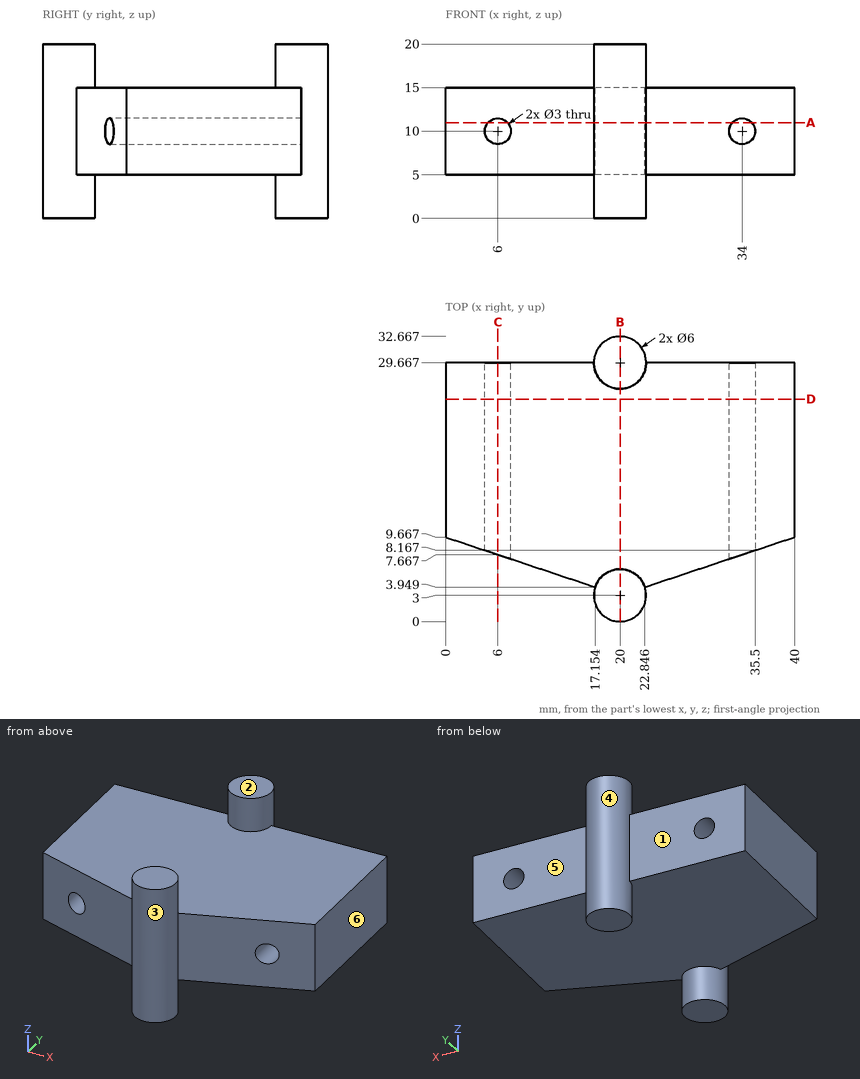
Can you work these out from the drawing? Everything is in mm from the part's minimum corner. A direction names the side the tool comes from. Coordinates: 2 decimals unless noted, no trailing zeros. Loops run counter-clockwise (first coordinate to the right, second up) from the corner with the lowest first, then second, coordinate; pieces in that order, holes last. Notation, with made-up numbers: (-36.75, -8.5) - (10.25, -8.5) arc R16 cw to (10.25, 18.5) - close; hole circle Ø6 at (65.5, 14.5). An arc over 180 degrees is marked (long way). Put each result on its own line as item: value. Start each with the question number.
Item 1: If we mould it in two halves opening along Y, with no side actions, what happens to the marked faces 1, 2 and 3? For each: +Y half, -Y half, draft (parallel to the pull), parting line (faces both ways), or undercut.
Item 2: If I drill on line 1 along X through (y, z) = (21.5, 10); line 2 along Z through (x, y) = (34, 18); line 3 along Z through (x, y) = (4, 9.5), over which ranges is the centre line in solid material (lowest first)?
Item 3: Suppose I cut it at A-A (z = 11). Please give me the cut outline in (x, y), and give its area (3 significant figures).
Item 4: Suppose I cut it at B-B (x = 20). Please give me the cut outline in (y, z).
Item 5: Which directions (+Z, -Z, +X, -X, +Y, -Y) give clear straight access to the entire face, cutting with the end or side of a thin tool? Please do the marked faces 4, 5 and 6.
Item 6: For pin 1 (11 mm diameter, centred on x = 6, z = 9, fed in from +Y); pin 2 (10 mm diameter, centred on x = 13.5, z = 16, fed in from +Y) (1 decimal); pin 3 (12 mm diameter, centred on x = 26, y = 13, fed in from -Z), each with a flat end and sliding along its axis, tell me the tip position at first contact or that it passes through.
Item 7: Suppose I cut it at C-C (x = 6). Please give me the cut outline in (y, z), and give its area (3 significant figures).
Item 8: Suppose I cut it at D-D (y = 25.5). Please give me the cut outline in (x, z).
Here are the results:
1. face 1: +Y half
1. face 2: draft
1. face 3: undercut
2. line 1: 0 to 4.5, 7.5 to 32.5, 35.5 to 40
2. line 2: 5 to 8.5, 11.5 to 15
2. line 3: 5 to 15
3. outline: (0, 9.67) - (4.88, 8.04) - (4.88, 29.67) - (0, 29.67) - close; (7.12, 7.29) - (17.15, 3.95) arc R3 ccw (long way) to (22.85, 3.95) - (32.88, 7.29) - (32.88, 29.67) - (23, 29.67) arc R3 ccw to (17, 29.67) - (7.12, 29.67) - close; (35.12, 8.04) - (40, 9.67) - (40, 29.67) - (35.12, 29.67) - close
3. area: 866 mm²
4. outline: (0, 0) - (6, 0) - (6, 5) - (26.67, 5) - (26.67, 0) - (32.67, 0) - (32.67, 20) - (26.67, 20) - (26.67, 15) - (6, 15) - (6, 20) - (0, 20) - close
5. face 4: none
5. face 5: +Z, -Z, +X, +Y
5. face 6: +Z, -Z, +X, +Y, -Y
6. pin 1: y = 29.67
6. pin 2: y = 32.3
6. pin 3: z = 5
7. outline: (7.67, 5) - (29.67, 5) - (29.67, 8.5) - (7.67, 8.5) - close; (7.67, 11.5) - (29.67, 11.5) - (29.67, 15) - (7.67, 15) - close
7. area: 154 mm²
8. outline: (0, 5) - (40, 5) - (40, 15) - (0, 15) - close; hole circle Ø3 at (6, 10); hole circle Ø3 at (34, 10)
